Geometry: see drawing. Coordinates: mm, zero at the bounding-box minimum. A direction names the side the tool comes from. Give positions to 0.01 mm unless a question says otherwise; leave off trailing zeros. Loops run counter-clockwise (first coordinate to the right, second up) from the corner with the lowest first, then second, coordinate; pieces in that order, holes last. Notation, with made-up numbers: (87, 81.25) -> (98, 81.25) arc R5 cw to (98, 85.25) -> close; hole circle Ø7 at (-2, 1). An arc over 180 degrees is marked (long way). One line per question, with ' | ' between items.
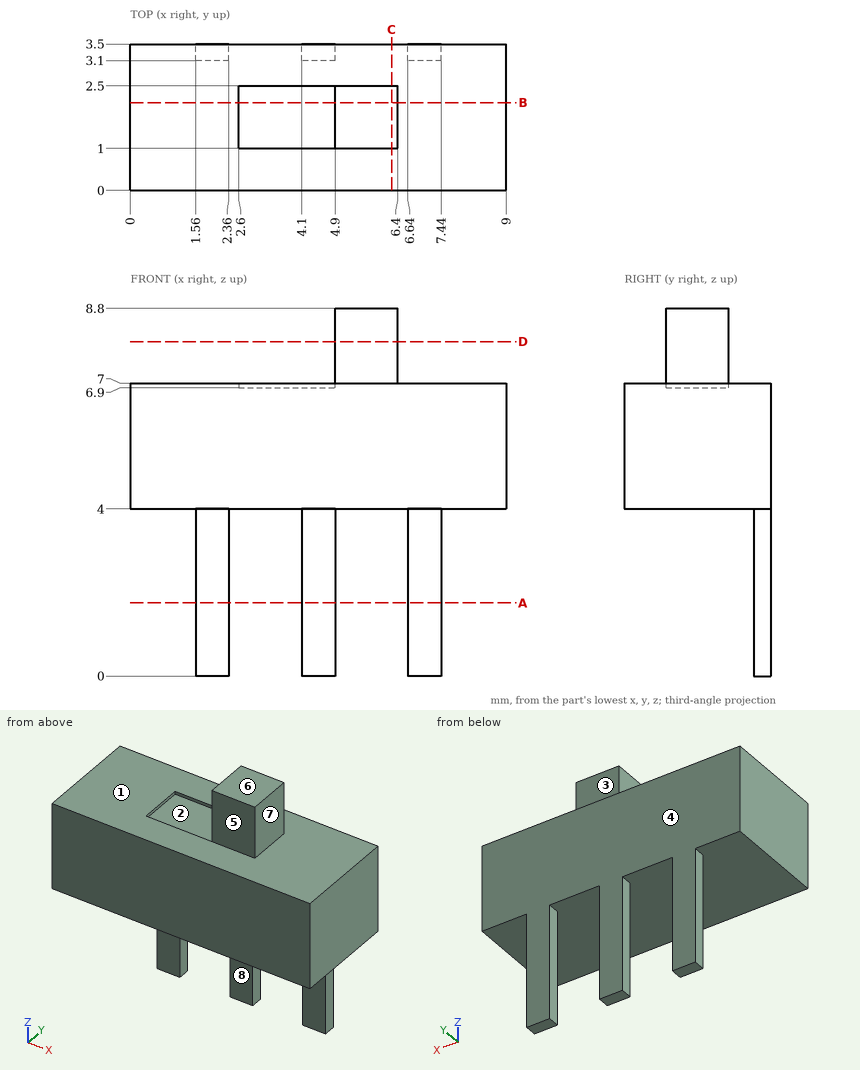
1. Section query D-D (z = 8). Output: boundary loops of the cut face in (x, y), then the cut area to 3 significant figures.
Determined:
outline: (4.9, 1) -> (6.4, 1) -> (6.4, 2.5) -> (4.9, 2.5) -> close | area: 2.25 mm2
2. Section query A-A (z = 1.75). Output: boundary loops of the cut face in (x, y).
Determined:
outline: (1.56, 3.1) -> (2.36, 3.1) -> (2.36, 3.5) -> (1.56, 3.5) -> close; (4.1, 3.1) -> (4.9, 3.1) -> (4.9, 3.5) -> (4.1, 3.5) -> close; (6.64, 3.1) -> (7.44, 3.1) -> (7.44, 3.5) -> (6.64, 3.5) -> close
3. Pull-direction query (Y, two-part tool) for the marked faces 1, 2 and 3; classes: pulls with the +Y half, pulls with the -Y half, needs draft (parallel to the pull), parting line crosses it, or undercut.
Determined:
face 1: needs draft | face 2: undercut | face 3: pulls with the +Y half
4. Section query B-B (y = 2.1). Output: boundary loops of the cut face in (x, z), then the cut area to 3 significant figures.
Determined:
outline: (0, 4) -> (9, 4) -> (9, 7) -> (6.4, 7) -> (6.4, 8.8) -> (4.9, 8.8) -> (4.9, 6.9) -> (2.6, 6.9) -> (2.6, 7) -> (0, 7) -> close | area: 29.5 mm2
5. Pin query (flat end, axial travel): P1, Ø1, axis at x = 4, y = 2, coming from the -Z side; P2, Ø0.8, axis at y = 2, z = 8, coming from the +X side; P3, Ø1.6, axis at x = 5.5, z = 8, coming from the -Y side. Return the tip coordinate at first contact, or that it passes through.
Determined:
P1: stops at z = 4 | P2: stops at x = 6.4 | P3: stops at y = 1
6. Ray query, line 1 along X through (y, z) = (3.3, 2); line 2 along Z through (x, y) = (5, 1.3); line 3 along X through (y, z) = (2.4, 8.25). Return the intervals inside material, ascending. Write a range as from..to.
Determined:
line 1: x = 1.56..2.36, 4.1..4.9, 6.64..7.44 | line 2: z = 4..8.8 | line 3: x = 4.9..6.4
7. Section query C-C (x = 6.25). Output: boundary loops of the cut face in (y, z).
Determined:
outline: (0, 4) -> (3.5, 4) -> (3.5, 7) -> (2.5, 7) -> (2.5, 8.8) -> (1, 8.8) -> (1, 7) -> (0, 7) -> close
8. Reachability of the marked faces 4, 5, 6, 7 and 8 from +Z, -Z, +X, -X, +Y, -Y: full face, straight path, thin tool, end or side. Return the list, or none.
Determined:
face 4: +Z, -Z, +X, -X, +Y | face 5: +Z, +X, -X, -Y | face 6: +Z, +X, -X, +Y, -Y | face 7: +Z, +X, +Y, -Y | face 8: -Z, +X, -X, -Y
